Work out the finished part from the listing and answer in its coordinate system (mm). A direction names the side the tool comes from. Round coordinates to 2 decimals unless told otherwise and drop trailing zeros. Loops run counter-clockwise (first coordinate to the right, second up) from the corner with the lowest first, then second, coordinate; pieces in that order, holes last.
```python
from build123d import *

# Parameters (mm, degrees)
SKETCH1_W            = 46
SKETCH1_H            = 44
BOSS_EXTRUDE1_DEPTH  = 32
SKETCH2_R            = 2.65
CUT_EXTRUDE1_DEPTH   = 46.133136386
LPATTERN1_COUNT      = 2
LPATTERN1_PITCH      = 26
LPATTERN1_COUNT_DIR2 = 2
LPATTERN1_PITCH_DIR2 = 28
SKETCH3_R            = 11
CUT_EXTRUDE2_DEPTH   = 7
FILLET1_R            = 2
SKETCH4_R            = 4.5
CUT_EXTRUDE3_DEPTH   = 22
LPATTERN2_COUNT      = 2
LPATTERN2_PITCH      = 28
LPATTERN2_COUNT_DIR2 = 2
LPATTERN2_PITCH_DIR2 = 26
SKETCH5_R            = 5
CUT_EXTRUDE4_DEPTH   = 46.133136386


with BuildPart() as part:
    # Sketch1 → Boss-Extrude1 (new body)
    with BuildSketch(Plane(origin=(0, 0, 0), x_dir=(1, 0, 0), z_dir=(0, 1, 0))):
        Rectangle(SKETCH1_W, SKETCH1_H)
    extrude(amount=BOSS_EXTRUDE1_DEPTH)

    # Sketch2 → Cut-Extrude1 (cut, through all)
    with BuildSketch(Plane.XZ):
        with Locations(Location((-14, -13, 0), (0, 0, 270))):
            Circle(SKETCH2_R)
    cut_extrude1 = extrude(amount=-CUT_EXTRUDE1_DEPTH, mode=Mode.SUBTRACT)

    # LPattern1: Cut-Extrude1 2 × 2
    with Locations(*[(j * LPATTERN1_PITCH_DIR2, 0, i * LPATTERN1_PITCH) for i in range(LPATTERN1_COUNT) for j in range(LPATTERN1_COUNT_DIR2) if (i, j) != (0, 0)]):
        add(cut_extrude1, mode=Mode.SUBTRACT)

    # Sketch3 → Cut-Extrude2 (cut)
    with BuildSketch(Plane(origin=(0, 32, 0), x_dir=(1, 0, 0), z_dir=(0, 1, 0))):
        with Locations(Location((0, 0, 0), (0, 0, 270))):
            Circle(SKETCH3_R)
    extrude(amount=-CUT_EXTRUDE2_DEPTH, mode=Mode.SUBTRACT)

    # Fillet1
    fillet1_edges = [part.edges().sort_by_distance(p)[0] for p in [
        (-23, 32, 0),
        (0, 32, 22),
        (23, 32, 0),
        (23, 16, 22),
        (-23, 16, 22),
        (-23, 16, -22),
        (23, 16, -22),
        (0, 32, -22),
    ]]
    fillet(fillet1_edges, radius=FILLET1_R)

    # Sketch4 → Cut-Extrude3 (cut)
    with BuildSketch(Plane(origin=(0, 32, 0), x_dir=(1, 0, 0), z_dir=(0, 1, 0))):
        with Locations(Location((14, -13, 0), (0, 0, 270))):
            Circle(SKETCH4_R)
    cut_extrude3 = extrude(amount=-CUT_EXTRUDE3_DEPTH, mode=Mode.SUBTRACT)

    # LPattern2: Cut-Extrude3 2 × 2
    with Locations(*[(-i * LPATTERN2_PITCH, 0, -j * LPATTERN2_PITCH_DIR2) for i in range(LPATTERN2_COUNT) for j in range(LPATTERN2_COUNT_DIR2) if (i, j) != (0, 0)]):
        add(cut_extrude3, mode=Mode.SUBTRACT)

    # Sketch5 → Cut-Extrude4 (cut, through all)
    with BuildSketch(Plane(origin=(0, 32, 0), x_dir=(1, 0, 0), z_dir=(0, 1, 0))):
        with Locations(Location((0, 0, 0), (0, 0, 270))):
            Circle(SKETCH5_R)
    extrude(amount=-CUT_EXTRUDE4_DEPTH, mode=Mode.SUBTRACT)


solid = part.part
```
1. Consider probe 1 along X at (y, z) = (16, -13); probe 2 along X at (y, z) = (5.5, 13); probe 3 along Z at (x, y) = (17.5, 24.5). Determine where each line is inside the solid, lowest interval first.
Answer key:
probe 1: x = -23 to -18.5, -9.5 to 9.5, 18.5 to 23
probe 2: x = -23 to -16.65, -11.35 to 11.35, 16.65 to 23
probe 3: z = -22 to -15.83, -10.17 to 10.17, 15.83 to 22
2. Given pin 1 (7 mm diameter, centred on x = -14, z = 13, fed in from +Y); pin 2 (4 mm diameter, centred on x = 14, z = 13, fed in from -Y) (3 decimals), each flat-ended and moving along its own axis, determine where each tip first touches the part or whether it passes through.
Answer key:
pin 1: stops at y = 10
pin 2: passes through
3. Determine the mould class of faces 3 (the face through (-16, 10, 15)), 4 (the face through (-22.43, 15.21, 21.4)), 5 (the face through (-22.43, 15.21, -21.4)), 6 (the face through (12, 10, 15)) for opening direction Z: +Z half, -Z half, draft (parallel to the pull), parting line (faces both ways), or undercut.
Answer key:
face 3: undercut
face 4: +Z half
face 5: -Z half
face 6: undercut
4. Find section A-A (z = 13). Write down the section's boundary in (x, y), then the cut area to 3 significant figures.
Answer key:
outline: (-23, 0) - (-16.65, 0) - (-16.65, 10) - (-18.5, 10) - (-18.5, 32) - (-21, 32) arc R2 ccw to (-23, 30) - close; (-11.35, 0) - (11.35, 0) - (11.35, 10) - (9.5, 10) - (9.5, 32) - (-9.5, 32) - (-9.5, 10) - (-11.35, 10) - close; (16.65, 0) - (23, 0) - (23, 30) arc R2 ccw to (21, 32) - (18.5, 32) - (18.5, 10) - (16.65, 10) - close
area: 968 mm2
5. Which of the six approach directions +Z, -Z, +X, -X, +Y, -Y give full straight-line access (tool end or side, diameter ignored) to faces 1 (the face through (-10.74, 28.55, -2.38)), 2 (the face through (-22.43, 31.4, -0.28))?
Answer key:
face 1: +Y
face 2: +Z, -Z, -X, +Y
6. Find section C-C (x = -14). Write down the section's boundary in (y, z).
Answer key:
outline: (0, -22) - (30, -22) arc R2 ccw to (32, -20) - (32, -17.5) - (10, -17.5) - (10, -15.65) - (0, -15.65) - close; (0, -10.35) - (10, -10.35) - (10, -8.5) - (32, -8.5) - (32, 8.5) - (10, 8.5) - (10, 10.35) - (0, 10.35) - close; (0, 15.65) - (10, 15.65) - (10, 17.5) - (32, 17.5) - (32, 20) arc R2 ccw to (30, 22) - (0, 22) - close
7. Find section B-B (y = 24). Write down the section's boundary in (x, z).
Answer key:
outline: (-23, -20) arc R2 ccw to (-21, -22) - (21, -22) arc R2 ccw to (23, -20) - (23, 20) arc R2 ccw to (21, 22) - (-21, 22) arc R2 ccw to (-23, 20) - close; hole circle Ø9 at (-14, -13); hole circle Ø9 at (-14, 13); hole circle Ø10 at (0, 0); hole circle Ø9 at (14, -13); hole circle Ø9 at (14, 13)
8. Find section D-D (z = 0). Write down the section's boundary in (x, y).
Answer key:
outline: (-23, 0) - (-5, 0) - (-5, 25) - (-11, 25) - (-11, 32) - (-21, 32) arc R2 ccw to (-23, 30) - close; (5, 0) - (23, 0) - (23, 30) arc R2 ccw to (21, 32) - (11, 32) - (11, 25) - (5, 25) - close
